Read the model definition and answer for the solid it produces. Units are mm, in the model's axes. Face numbers are marked on the shaded views. Coordinates: 2 decimals unless noted, no trailing zeros. Write each loop counter-clockwise with the first axis right and the second up, starting at its lowest first coordinate (ties: lowest second). Pieces come first, ordered by that corner, then holes. Notation, with made-up numbers: (-21.5, 79.25) - (25.5, 79.25) arc R19 ccw to (25.5, 108.25) - close; hole circle Ø2 at (78.5, -36.75). An arc over 180 degrees is marked (long way). Use a Markdown table: item, result.
from build123d import *

# Parameters (mm, degrees)
F1_DEPTH = 31.75
F3_D     = 5.4102


with BuildPart() as f1:
    # F0 (on Front) → F1 (new body)
    with BuildSketch(Plane.XZ):
        with BuildLine():
            Line((159.1974866311, 85.2424), (110.2795238258, 62.4315793225))
            ThreePointArc((110.2795238258, 62.4315793225), (63.4585527357, 16.521426637), (0, 0))
            ThreePointArc((0, 0), (73.6360318528, -25.8222553056), (118.37924, -89.7526814014))
            Line((118.37924, -89.7526814014), (270.77924, -89.7526814014))
            Line((270.77924, -89.7526814014), (270.77924, 18.1973185986))
            Line((270.77924, 18.1973185986), (159.1974866311, 85.2424))
        make_face()
    extrude(amount=F1_DEPTH)

    # F3 (through all)
    with Locations(Plane.XZ.offset(31.75)):
        with Locations((143.77924, -38.9526814014), (219.97924, -38.9526814014)):
            Hole(F3_D / 2)


solid = f1.part
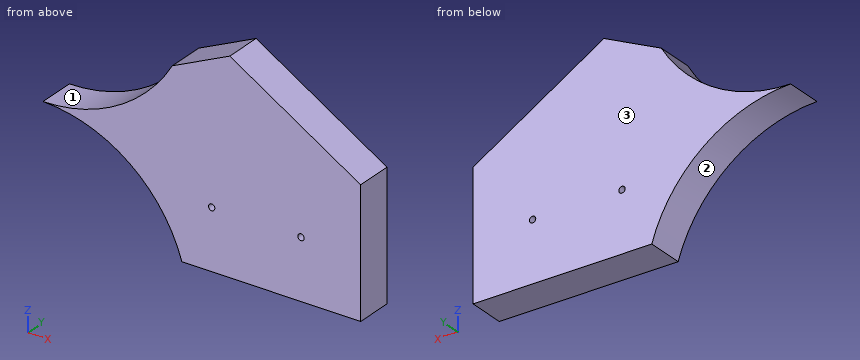
(1) A cutting plane is placed at C-C, the plane x = 47. Write down the section's boundary in (y, z).
Report:
| item | result |
|---|---|
| outline | (-31.75, -10.31) - (0, -10.31) - (0, 8.7) - (-31.75, 8.7) - close |
(2) Each of these flat-tipped pins is pushed along its axis until it touches: P1, Ø2, axis at x = 36.5, y = -23.5, coming from the +Z side; P2, Ø1, axis at y = -17, z = 39, coming from the +X side. Where does it stop, or does it pass through?
Report:
| item | result |
|---|---|
| P1 | stops at z = 5.42 |
| P2 | stops at x = 236.99 |
(3) Straight lines are drawn through the part: L1, parallel to Z at x = 218.5, y = -15; L2, parallel to X at y = -18, z = 75.5; L3, parallel to Z at x = 236, y = -2.5. For each, find the intervals that lie inside material, in ascending order.
Report:
| item | result |
|---|---|
| L1 | z = -89.75 to -41.22, -36.69 to 49.61 |
| L2 | x = 138.3 to 175.41 |
| L3 | z = -89.75 to 39.09 |
(4) A cutting plane is placed at A-A, the plane y = -25. Write down the section's boundary in (x, z).
Report:
| item | result |
|---|---|
| outline | (0, 0) arc R127.33 cw to (118.38, -89.75) - (270.78, -89.75) - (270.78, 18.2) - (159.2, 85.24) - (110.28, 62.43) arc R127.33 cw to start; hole circle Ø5.41 at (143.78, -38.95); hole circle Ø5.41 at (219.98, -38.95) |
(5) The mould has two halves that part along Z. Classify the marked faces 1, 2 and 3: pulls with the +Z half, pulls with the -Z half, needs draft (parallel to the pull), parting line crosses it, or undercut.
Report:
| item | result |
|---|---|
| face 1 | pulls with the +Z half |
| face 2 | pulls with the -Z half |
| face 3 | needs draft |
(6) A cutting plane is placed at B-B, the plane z = 73. Write down the section's boundary in (x, y), and give its area (3 significant figures).
Report:
| item | result |
|---|---|
| outline | (132.94, -31.75) - (179.57, -31.75) - (179.57, 0) - (132.94, 0) - close |
| area | 1,480 mm² |
